from build123d import *

# Parameters (mm, degrees)
SKETCH1_W           = 152.4
SKETCH1_H           = 152.4
BOSS_EXTRUDE1_DEPTH = 3.4036
SKETCH2_R           = 8.10895
CUT_EXTRUDE1_DEPTH  = 216.553020143
SKETCH3_W           = 50.8
SKETCH3_H           = 19.05
BOSS_EXTRUDE2_DEPTH = 19.05
SKETCH4_W           = 43.9928
SKETCH4_H           = 21.9964
CUT_EXTRUDE2_DEPTH  = 217.692602903
DRAFT1_ANGLE        = 15


with BuildPart() as part:
    # Sketch1 → Boss-Extrude1 (new body)
    with BuildSketch(Plane(origin=(0, 0, 0), x_dir=(1, 0, 0), z_dir=(0, 1, 0))):
        with Locations((76.2, 76.2)):
            Rectangle(SKETCH1_W, SKETCH1_H)
    extrude(amount=BOSS_EXTRUDE1_DEPTH)

    # Sketch2 → Cut-Extrude1 (cut, through all)
    with BuildSketch(Plane(origin=(0, 3.4036, 0), x_dir=(1, 0, 0), z_dir=(0, 1, 0))):
        with Locations(Location((63.5, 31.75, 0), (0, 0, 270))):
            Circle(SKETCH2_R)
        with Locations(Location((85.1154, 31.75, 0), (0, 0, 270))):
            Circle(SKETCH2_R)
    extrude(amount=-CUT_EXTRUDE1_DEPTH, mode=Mode.SUBTRACT)

    # Sketch3 → Boss-Extrude2 (add)
    with BuildSketch(Plane(origin=(0, 3.4036, 0), x_dir=(1, 0, 0), z_dir=(0, 1, 0))):
        with Locations((76.2, 53.975)):
            Rectangle(SKETCH3_W, SKETCH3_H)
    extrude(amount=BOSS_EXTRUDE2_DEPTH)

    # Sketch4 → Cut-Extrude2 (cut, through all)
    with BuildSketch(Plane(origin=(0, 22.4536, 0), x_dir=(1, 0, 0), z_dir=(0, 1, 0))):
        with Locations((76.2, 58.8518)):
            Rectangle(SKETCH4_W, SKETCH4_H)
    extrude(amount=-CUT_EXTRUDE2_DEPTH, mode=Mode.SUBTRACT)

    # Draft1
    draft1_faces = [part.faces().sort_by_distance(p)[0] for p in [
        (54.2036, 10.674787523, -56.314190406),
        (98.1964, 10.674787523, -56.314190406),
        (76.2, 11.2268, -47.8536),
    ]]
    draft(draft1_faces, Plane.ZX.offset(22.4536), DRAFT1_ANGLE)


solid = part.part
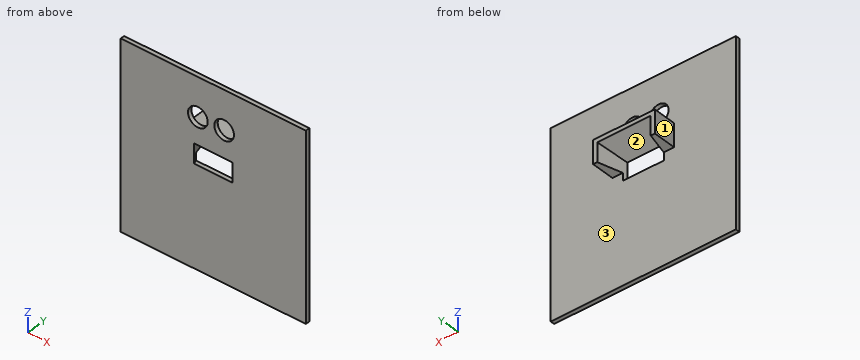
The listing builds one solid part. Answer for the finished solid, in the listing's coordinates (mm). Face numbers are marked on the shaded views. Coordinates: 2 decimals unless noted, no trailing zeros. Loops run counter-clockwise (first coordinate to the right, second up) from the corner with the lowest first, then second, coordinate; pieces in that order, holes last.
1) Find section B-B on x = 63.5. Write down the section's boundary in (y, z), then the cut area to 3 significant figures.
2) Flat-ended cylindrical pins translate along their axes: pin 1 Ø9.5 at (x, y) = (97, 10.5) entering from -Z; pin 2 Ø9.5 at (y, z) = (17, -56) entering from +X; pin 3 Ø1.5 at (x, y) = (59, 10) entering from +Z; pin 4 Ø14.5 at (x, z) = (63.5, -31.75) entering from +Y. Find the tip coordinate at first contact, or state that the pin passes through.
3) Find the intervals of material crossed by L1, parallel to X at y = 2.4, z = -31.75; L2, parallel to Y at x = 18, z = -13; L3, parallel to Z at x = 58, y = 2.5, in increasing order.
4) Find section A-A on z = -60. Write down the section's boundary in (x, y).
5) Find section C-C on z = -31.75. Write down the section's boundary in (x, y), then the cut area to 3 significant figures.
6) Determine the mould class of the marked faces 1, 2 and 3 for opening direction X: pulls with the +X half, pulls with the -X half, needs draft (parallel to the pull), parting line crosses it, or undercut.
7) Find section D-D on y = 6.5. Write down the section's boundary in (x, z), then the cut area to 3 significant figures.
Values:
1. outline: (0, -152.4) - (3.4, -152.4) - (3.4, -69.85) - (0, -69.85) - close; (0, -53.87) - (22.45, -47.85) - (22.45, -44.45) - (3.4, -44.45) - (3.4, -39.86) - (0, -39.86) - close; (0, -23.64) - (3.4, -23.64) - (3.4, 0) - (0, 0) - close
1. area: 521 mm2
2. pin 1: stops at z = -63.5
2. pin 2: stops at x = 101.6
2. pin 3: stops at z = -44.45
2. pin 4: passes through
3. L1: x = 0 to 55.39, 71.61 to 77.01, 93.22 to 152.4
3. L2: y = 0 to 3.4
3. L3: z = -152.4 to -37.71, -25.79 to 0
4. outline: (0, 0) - (60.22, 0) - (54.2, 22.45) - (50.8, 22.45) - (50.8, 3.4) - (0, 3.4) - close; (92.18, 0) - (152.4, 0) - (152.4, 3.4) - (101.6, 3.4) - (101.6, 22.45) - (98.2, 22.45) - close
5. outline: (0, 0) - (55.39, 0) - (55.39, 3.4) - (0, 3.4) - close; (71.61, 0) - (77.01, 0) - (77.01, 3.4) - (71.61, 3.4) - close; (93.22, 0) - (152.4, 0) - (152.4, 3.4) - (93.22, 3.4) - close
5. area: 408 mm2
6. face 1: pulls with the -X half
6. face 2: undercut
6. face 3: needs draft
7. outline: (50.8, -63.5) - (58.48, -63.5) - (58.48, -52.13) - (93.92, -52.13) - (93.92, -63.5) - (101.6, -63.5) - (101.6, -44.45) - (50.8, -44.45) - close
7. area: 565 mm2
